Here's how the part is built. I have some questions about the finished solid (model axes, mm). A direction names the side the tool comes from. Coordinates: 2 decimals unless noted, no trailing zeros. Write each loop counter-clockwise with the first axis right and the second up, starting at its lowest first coordinate (ties: lowest second). Pieces come first, ordered by that corner, then holes. Notation, with made-up numbers: (47.25, 31.25) -> (81.25, 31.25) arc R14 ccw to (81.25, 44.25) -> close; hole circle Ø5 at (-38.75, 39). An arc over 180 degrees is marked (long way). Use a Markdown table: item, result. Add a question column.
Autodesk Inventor part; units mm, degrees
ref_plane "YZ Plane" through (0, 0, 0) normal (1, 0, 0) x (0, 1, 0)
ref_plane "XZ Plane" through (0, 0, 0) normal (0, 1, 0) x (-1, 0, 0)
ref_plane "XY Plane" through (0, 0, 0) normal (0, 0, 1) x (1, 0, 0)
sketch "Sketch1" plane through (0, 0, 0) normal (0, 1, 0) x (-1, 0, 0)
  line L0 (0, 0) -> (-130, 0)
  line L1 (-130, 0) -> (-130, -120)
  line L2 (-130, -120) -> (0, -120)
  line L3 (0, -120) -> (0, 0)
  dimension "d0" = 130
  dimension "d1" = 120
extrude "Extrusion1" add sketch "Sketch1" along normal blind 25
sketch "Sketch2" plane through (0, 0, 0) normal (0, -1, 0) x (1, 0, 0)
  line L0 (110, -6.6572) -> (20, -6.6572)
  line L1 (20, -6.6572) -> (20, -110)
  line L2 (20, -110) -> (110, -110)
  line L3 (110, -110) -> (110, -6.6572)
  line L4 (0, -120) -> (0, 0)
  line L5 (0, 0) -> (130, 0)
  line L6 (130, -120) -> (0, -120)
  line L7 (130, 0) -> (130, -120)
  dimension "d5" = 6.6572
  dimension "d46" = 20
  dimension "d47" = 20
  dimension "d48" = 10
extrude "Extrusion2" cut sketch "Sketch2" against normal blind 22 contours L3 L2 L1 L0
sketch "Sketch4" plane through (0, 22, 0) normal (0, -1, 0) x (1, 0, 0)
  line L0 (130, -120) -> (0, -120)
  line L1 (40, -90) -> (50, -90)
  line L2 (50, -90) -> (50, -80)
  line L3 (50, -80) -> (40, -80)
  line L4 (40, -80) -> (40, -90)
  line L5 (0, -120) -> (0, 0)
  line L6 (20, -110) -> (20, -6.6572)
  line L7 (110, -110) -> (20, -110)
  dimension "d42" = 10
  dimension "d43" = 10
  dimension "d49" = 20
  dimension "d50" = 20
extrude "Extrusion3" cut sketch "Sketch4" against normal blind 22
sketch "Sketch5" plane through (0, 0, 0) normal (0, 0, 1) x (1, 0, 0)
  line L0 (20, 22) -> (110, 22)
  line L1 (110, 22) -> (110, 0)
  line L2 (110, 0) -> (20, 0)
  line L3 (20, 0) -> (20, 22)
  line L4 (0, 0) -> (0, 25)
  line L5 (130, 0) -> (130, 25)
  line L6 (0, 0) -> (130, 0)
  line L7 (130, 25) -> (0, 25)
  dimension "d13" = 20
  dimension "d14" = 20
  dimension "d15" = 0
  dimension "d16" = 3
extrude "Extrusion4" cut sketch "Sketch5" against normal blind 22 contours L0 L1 L2 L3
sketch "Sketch10" plane through (0, 0, 0) normal (0, -1, 0) x (1, 0, 0)
  circle A0 centre (10, -10) radius 4.7625
  line L0 (0, 0) -> (20, 0)
  line L1 (0, -120) -> (0, 0)
  dimension "d51" = 10
  dimension "d52" = 10
  dimension "d53" = 9.525
ref_plane "Work Plane3" through (65, 0, 0) normal (1, 0, 0) x (0, 0, -1)
ref_plane "Work Plane4" through (0, 25, -60) normal (0, 0, 1) x (1, 0, 0)
extrude "Extrusion7" cut sketch "Sketch10" against normal blind 25
mirror "Mirror4" about plane through (0, 25, -60) normal (0, 0, 1) of "Extrusion7"
mirror "Mirror5" about plane through (65, 0, 0) normal (1, 0, 0) of "Extrusion7", "Mirror4"
properties part number "Case_Top_Partv1"
Q1. Thinking about a two-plate mould opening in Z: for faces 1 (the flat face through (110, 11, -54)), 2 (the flat face through (50, 23, -85)), 3 (the cylindrical face through (124.758, 12.325, -10.209)), 4 (the flat face through (64, 11, -110)), which applies, released by +Z, released by -Z, zero draft, split by the parting line, or undercut?
Q2. Suppose I cut it at C-C, the plane x = 10. Write out the boundary of the cut face in (y, z).
Q3. Suppose I cut it at B-B, the plane y = 14.25. Write out the boundary of the cut face in (x, z) (1 decimal), and give its area (3 significant figures).
Q4. Suppose I cut it at A-A, the plane z = -10. Write out the boundary of the cut face in (x, y).
Q5. Please list where these lines run through material, in increasing order: line 1 (Z direction, x = 120, y = 12); line 2 (X direction, y = 17.5, z = -91); line 3 (X direction, y = 5.5, z = -109).
Q6. Which directions (+Z, -Z, +X, -X, +Y, -Y) give clear straight access to the entire face, cutting with the end or side of a thin tool? Please do faces 5 (the flat face through (64, 22, -54)), 6 (the flat face through (66, 12, -120)), 7 (the flat face through (45, 23, -90)).
Q7. Will these pins go through, and if not, where does the flat tip stop? pin 1 (6 mm diameter, centred on x = 55, y = 17, fed in from +Z); pin 2 (1.5 mm diameter, centred on x = 64, z = -85.5, fed in from -Y).
Q8. Suppose I cut it at D-D, the plane z = -62. Write out the boundary of the cut face in (x, y), and give its area (3 significant figures).
Answer key:
| question | item | result |
|---|---|---|
| 1 | face 1 | zero draft |
| 1 | face 2 | undercut |
| 1 | face 3 | undercut |
| 1 | face 4 | released by +Z |
| 2 | outline | (0, -120) -> (25, -120) -> (25, -114.76) -> (0, -114.76) -> close; (0, -105.24) -> (25, -105.24) -> (25, -14.76) -> (0, -14.76) -> close; (0, -5.24) -> (25, -5.24) -> (25, 0) -> (0, 0) -> close |
| 3 | outline | (0, -120) -> (130, -120) -> (130, 0) -> (110, 0) -> (110, -110) -> (20, -110) -> (20, 0) -> (0, 0) -> close; hole circle Ø9.5 at (10, -110); hole circle Ø9.5 at (10, -10); hole circle Ø9.5 at (120, -110); hole circle Ø9.5 at (120, -10) |
| 3 | area | 5,410 mm^2 |
| 4 | outline | (0, 0) -> (5.24, 0) -> (5.24, 25) -> (0, 25) -> close; (14.76, 0) -> (20, 0) -> (20, 22) -> (110, 22) -> (110, 0) -> (115.24, 0) -> (115.24, 25) -> (14.76, 25) -> close; (124.76, 0) -> (130, 0) -> (130, 25) -> (124.76, 25) -> close |
| 5 | line 1 | z = -120 to -114.76, -105.24 to -14.76, -5.24 to 0 |
| 5 | line 2 | x = 0 to 20, 110 to 130 |
| 5 | line 3 | x = 0 to 5.34, 14.66 to 20, 110 to 115.34, 124.66 to 130 |
| 6 | face 5 | +Z, -Y |
| 6 | face 6 | -Z, +X, -X, +Y, -Y |
| 6 | face 7 | +Y, -Y |
| 7 | pin 1 | stops at z = -110 |
| 7 | pin 2 | stops at y = 22 |
| 8 | outline | (0, 0) -> (20, 0) -> (20, 22) -> (110, 22) -> (110, 0) -> (130, 0) -> (130, 25) -> (0, 25) -> close |
| 8 | area | 1,270 mm^2 |
